```python
from build123d import *
from build123d.topology import SkipClean

# Parameters (mm, degrees)
SKETCH9_W            = 36
SKETCH9_H            = 36
BOSS_EXTRUDE1_DEPTH  = 40
CHAMFER2_SIZE        = 18
SKETCH10_W           = 36
SKETCH10_H           = 40
BOSS_EXTRUDE2_DEPTH  = 8
SKETCH12_W           = 44
SKETCH12_H           = 40
BOSS_EXTRUDE3_DEPTH  = 8
CHAMFER3_SIZE        = 18
CHAMFER4_SIZE        = 6
SKETCH13_W           = 36.769552622
SKETCH13_H           = 20
CUT_EXTRUDE6_DEPTH   = 39.59798
SKETCH22_R           = 2.1
CUT_EXTRUDE13_DEPTH  = 6
BOSS_EXTRUDE7_DEPTH  = 8
BOSS_EXTRUDE8_DEPTH  = 12
BOSS_EXTRUDE9_DEPTH  = 4
CUT_EXTRUDE14_DEPTH  = 4
CUT_EXTRUDE15_DEPTH  = 4
SKETCH28_W           = 4
SKETCH28_H           = 28
CUT_EXTRUDE16_DEPTH  = 77.210235533
BOSS_EXTRUDE11_DEPTH = 28
SKETCH31_W           = 10
SKETCH31_H           = 36
CUT_EXTRUDE17_DEPTH  = 22
SKETCH32_W           = 44
SKETCH32_H           = 18.026894841
CUT_EXTRUDE18_DEPTH  = 72.888803022
BOSS_EXTRUDE12_DEPTH = 10
BOSS_EXTRUDE13_DEPTH = 10
CHAMFER5_SIZE        = 6
CUT_EXTRUDE19_DEPTH  = 79.409183136
CHAMFER6_SIZE        = 6
SKETCH37_R           = 2.8
CUT_EXTRUDE20_DEPTH  = 7
BOSS_EXTRUDE14_DEPTH = 14
CHAMFER7_SIZE        = 14
CHAMFER8_SIZE        = 4
BOSS_EXTRUDE15_START = 7
SKETCH41_R           = 2.8
BOSS_EXTRUDE15_DEPTH = 7
BOSS_EXTRUDE16_START = 7
SKETCH42_R           = 2.8
BOSS_EXTRUDE16_DEPTH = 7
CHAMFER9_SIZE        = 1
SKETCH43_R           = 2.25
CUT_EXTRUDE21_DEPTH  = 69.381283989
SKETCH44_R           = 4
CUT_EXTRUDE22_DEPTH  = 7
CHAMFER11_SIZE       = 4
CHAMFER12_SIZE       = 3
SKETCH48_R           = 2.1
CUT_EXTRUDE26_DEPTH  = 4
SKETCH49_R           = 2.1
CUT_EXTRUDE27_DEPTH  = 4
CUT_EXTRUDE28_DEPTH  = 79.409183136


with BuildPart() as part:
    # Sketch9 → Boss-Extrude1 (new body)
    with BuildSketch(Plane(origin=(0, 0, 0), x_dir=(1, 0, 0), z_dir=(0, 1, 0))):
        with Locations((18, 18)):
            Rectangle(SKETCH9_W, SKETCH9_H)
    extrude(amount=BOSS_EXTRUDE1_DEPTH)

    # Chamfer2
    chamfer2_edges = [part.edges().sort_by_distance(p)[0] for p in [
        (0, 20, -36),
    ]]
    chamfer(chamfer2_edges, length=CHAMFER2_SIZE)

    # Sketch10 → Boss-Extrude2 (add)
    with BuildSketch(Plane(origin=(36, 0, 0), x_dir=(0, 0, -1), z_dir=(1, 0, 0))):
        with Locations((18, 20)):
            Rectangle(SKETCH10_W, SKETCH10_H)
    extrude(amount=BOSS_EXTRUDE2_DEPTH)

    # Sketch12 → Boss-Extrude3 (add)
    with BuildSketch(Plane.XY):
        with Locations((22, 20)):
            Rectangle(SKETCH12_W, SKETCH12_H)
    extrude(amount=BOSS_EXTRUDE3_DEPTH)

    # Chamfer3
    chamfer3_edges = [part.edges().sort_by_distance(p)[0] for p in [
        (44, 20, -36),
        (0, 20, 8),
    ]]
    chamfer(chamfer3_edges, length=CHAMFER3_SIZE)

    # Chamfer4
    chamfer4_edges = [part.edges().sort_by_distance(p)[0] for p in [
        (44, 20, 8),
    ]]
    chamfer(chamfer4_edges, length=CHAMFER4_SIZE)

    # Sketch13 → Cut-Extrude6 (cut)
    with BuildSketch(Plane(origin=(23, 0, 23), x_dir=(0.7071067811865465, 0, -0.7071067811865487), z_dir=(0.7071067811865487, 0, 0.7071067811865465))):
        with Locations((25.455844123, 22)):
            Rectangle(SKETCH13_W, SKETCH13_H)
    extrude(amount=-CUT_EXTRUDE6_DEPTH, mode=Mode.SUBTRACT)

    # Sketch22 → Cut-Extrude13 (cut)
    with BuildSketch(Plane(origin=(-9, 0, -9), x_dir=(-0.7071067811865487, 0, 0.7071067811865465), z_dir=(-0.7071067811865465, 0, -0.7071067811865487))):
        with Locations((-15.455844123, 36)):
            Circle(SKETCH22_R)
        with Locations((-35.455844123, 36)):
            Circle(SKETCH22_R)
        with Locations((-35.455844123, 4)):
            Circle(SKETCH22_R)
        with Locations((-15.455844123, 4)):
            Circle(SKETCH22_R)
    extrude(amount=-CUT_EXTRUDE13_DEPTH, mode=Mode.SUBTRACT)

    # Sketch23 → Boss-Extrude7 (add)
    with BuildSketch(Plane(origin=(0, 40, 0), x_dir=(1, 0, 0), z_dir=(0, 1, 0))):
        Polygon((26, 36), (44, 36), (44, 18), align=None)
    extrude(amount=-BOSS_EXTRUDE7_DEPTH)

    # Sketch24 → Boss-Extrude8 (add)
    with BuildSketch(Plane(origin=(0, 0, 0), x_dir=(-1, 0, 0), z_dir=(0, -1, 0))):
        Polygon((-44, 18), (-26, 36), (-44, 36), align=None)
    extrude(amount=-BOSS_EXTRUDE8_DEPTH)

    # Sketch25 → Boss-Extrude9 (add)
    with BuildSketch(Plane(origin=(0, 40, 0), x_dir=(1, 0, 0), z_dir=(0, 1, 0))):
        Polygon((18, -8), (38, -8), (44, -2), (44, 36), (18, 36), (0, 18), (0, 10), align=None)
    extrude(amount=BOSS_EXTRUDE9_DEPTH)

    # Sketch26 → Cut-Extrude14 (cut)
    with SkipClean():  # the faces are left unmerged after this step: merging them gives an invalid solid
        with BuildSketch(Plane(origin=(0, 32, 0), x_dir=(-1, 0, 0), z_dir=(0, -1, 0))):
            Polygon((-44, 36), (-44, -2), (-38, -8), (-18, -8), (0, 10), (-26, 36), align=None)
        extrude(amount=-CUT_EXTRUDE14_DEPTH, mode=Mode.SUBTRACT)

    # Sketch27 → Cut-Extrude15 (cut)
    with BuildSketch(Plane(origin=(0, 12, 0), x_dir=(1, 0, 0), z_dir=(0, 1, 0))):
        Polygon((44, -2), (44, 36), (26, 36), (0, 10), (18, -8), (38, -8), align=None)
    extrude(amount=-CUT_EXTRUDE15_DEPTH, mode=Mode.SUBTRACT)

    # Sketch28 → Cut-Extrude16 (cut, through all)
    with BuildSketch(Plane(origin=(0, 0, -36), x_dir=(-1, 0, 0), z_dir=(0, 0, -1))):
        with Locations((-24, 22)):
            Rectangle(SKETCH28_W, SKETCH28_H)
    extrude(amount=-CUT_EXTRUDE16_DEPTH, mode=Mode.SUBTRACT)

    # Sketch30 → Boss-Extrude11 (add)
    with BuildSketch(Plane(origin=(0, 8, 0), x_dir=(1, 0, 0), z_dir=(0, 1, 0))):
        Polygon((0, 10), (22, 10), (22, 32), align=None)
    extrude(amount=BOSS_EXTRUDE11_DEPTH)

    # Sketch31 → Cut-Extrude17 (cut)
    with BuildSketch(Plane(origin=(44, 0, 0), x_dir=(0, 0, -1), z_dir=(1, 0, 0))):
        with Locations((24, 22)):
            Rectangle(SKETCH31_W, SKETCH31_H)
    extrude(amount=-CUT_EXTRUDE17_DEPTH, mode=Mode.SUBTRACT)

    # Sketch32 → Cut-Extrude18 (cut, through all)
    with BuildSketch(Plane(origin=(0, 0, 0), x_dir=(-1, 0, 0), z_dir=(0, -1, 0))):
        with Locations((-22, 0.986552579)):
            Rectangle(SKETCH32_W, SKETCH32_H)
    extrude(amount=-CUT_EXTRUDE18_DEPTH, mode=Mode.SUBTRACT)

    # Sketch33 → Boss-Extrude12 (add)
    with BuildSketch(Plane(origin=(44, 0, 0), x_dir=(0, 0, -1), z_dir=(1, 0, 0))):
        Polygon((10, 8), (10, 0), (36, 0), (36, 8), (29, 8), (29, 4), (19, 4), (19, 8), align=None)
    extrude(amount=BOSS_EXTRUDE12_DEPTH)

    # Sketch35 → Boss-Extrude13 (add)
    with BuildSketch(Plane(origin=(44, 0, 0), x_dir=(0, 0, -1), z_dir=(1, 0, 0))):
        Polygon((10, 44), (10, 36), (19, 36), (19, 40), (29, 40), (29, 36), (36, 36), (36, 44), align=None)
    extrude(amount=BOSS_EXTRUDE13_DEPTH)

    # Chamfer5
    chamfer5_edges = [part.edges().sort_by_distance(p)[0] for p in [
        (54, 4, -10),
        (54, 4, -36),
        (54, 40, -10),
        (54, 40, -36),
    ]]
    chamfer(chamfer5_edges, length=CHAMFER5_SIZE)

    # Sketch36 → Cut-Extrude19 (cut, through all)
    with BuildSketch(Plane(origin=(0, 44, 0), x_dir=(1, 0, 0), z_dir=(0, 1, 0))):
        Polygon((14, 32), (14, 26), (10, 22), (4, 22), align=None)
    extrude(amount=-CUT_EXTRUDE19_DEPTH, mode=Mode.SUBTRACT)

    # Chamfer6
    chamfer6_edges = [part.edges().sort_by_distance(p)[0] for p in [
        (22, 22, -10),
    ]]
    chamfer(chamfer6_edges, length=CHAMFER6_SIZE)

    # Sketch37 → Cut-Extrude20 (cut)
    with BuildSketch(Plane(origin=(22, 0, 0), x_dir=(0, 0, -1), z_dir=(1, 0, 0))):
        with Locations(Location((24, 31, 0), (0, 0, 90))):
            Circle(SKETCH37_R)
        with Locations(Location((24, 13, 0), (0, 0, 90))):
            Circle(SKETCH37_R)
    extrude(amount=-CUT_EXTRUDE20_DEPTH, mode=Mode.SUBTRACT)

    # Sketch39 → Boss-Extrude14 (add)
    with BuildSketch(Plane.XY.offset(-10)):
        Polygon((48, 8), (16, 8), (16, 36), (48, 36), (48, 44), (0, 44), (0, 0), (48, 0), align=None)
    extrude(amount=BOSS_EXTRUDE14_DEPTH)

    # Chamfer7
    chamfer7_edges = [part.edges().sort_by_distance(p)[0] for p in [
        (48, 4, 4),
        (48, 40, 4),
    ]]
    chamfer(chamfer7_edges, length=CHAMFER7_SIZE - 0.0001)  # a hair under: the kernel refuses the full size

    # Chamfer8
    chamfer8_edges = [part.edges().sort_by_distance(p)[0] for p in [
        (17.00005, 0, 4),
        (0, 22, 4),
        (17.00005, 44, 4),
        (41.00005, 0, -2.99995),
        (48, 0, -9.99995),
        (51, 0, -13),
        (41.00005, 44, -2.99995),
        (48, 44, -9.99995),
        (51, 44, -13),
    ]]
    chamfer(chamfer8_edges, length=CHAMFER8_SIZE)

    # Sketch41 → Boss-Extrude15 (add)
    with BuildSketch(Plane(origin=(15, 0, 0), x_dir=(0, 0, -1), z_dir=(1, 0, 0)).offset(BOSS_EXTRUDE15_START)):
        with Locations((24, 31)):
            Circle(SKETCH41_R)
    extrude(amount=-BOSS_EXTRUDE15_DEPTH)

    # Sketch42 → Boss-Extrude16 (add)
    with BuildSketch(Plane(origin=(15, 0, 0), x_dir=(0, 0, -1), z_dir=(1, 0, 0)).offset(BOSS_EXTRUDE16_START)):
        with Locations((24, 13)):
            Circle(SKETCH42_R)
    extrude(amount=-BOSS_EXTRUDE16_DEPTH)

    # Chamfer9
    chamfer9_edges = [part.edges().sort_by_distance(p)[0] for p in [
        (54, 6, -29),
        (54, 4, -24),
        (54, 6, -19),
        (54, 38, -19),
        (54, 40, -24),
        (54, 38, -29),
    ]]
    chamfer(chamfer9_edges, length=CHAMFER9_SIZE - 0.0001)  # a hair under: the kernel refuses the full size

    # Sketch43 → Cut-Extrude21 (cut, through all)
    with BuildSketch(Plane(origin=(16, 0, 0), x_dir=(0, 0, -1), z_dir=(1, 0, 0))):
        with Locations(Location((3, 22, 0), (0, 0, 90))):
            Circle(SKETCH43_R)
    extrude(amount=-CUT_EXTRUDE21_DEPTH, mode=Mode.SUBTRACT)

    # Sketch44 → Cut-Extrude22 (cut)
    with BuildSketch(Plane.ZY):
        with Locations((-3, 22)):
            Circle(SKETCH44_R)
    extrude(amount=-CUT_EXTRUDE22_DEPTH, mode=Mode.SUBTRACT)

    # Chamfer10: read off the stored shape, not the designer's step
    # Chamfer10 outline → Chamfer10 (revolve, cut)
    with BuildSketch(Plane(origin=(0, 22, -3), x_dir=(0, 1, 0), z_dir=(0, 0, -1))):
        Polygon((8, 0), (4, 4), (4, 0), align=None)
    revolve(axis=Axis((0, 22, -3), (1, 0, 0)), mode=Mode.SUBTRACT)

    # Chamfer11
    chamfer11_edges = [part.edges().sort_by_distance(p)[0] for p in [
        (0, 44, -9),
    ]]
    chamfer(chamfer11_edges, length=CHAMFER11_SIZE)

    # Chamfer12
    chamfer12_edges = [part.edges().sort_by_distance(p)[0] for p in [
        (0, 0, -9),
    ]]
    chamfer(chamfer12_edges, length=CHAMFER12_SIZE)

    # Sketch48 → Cut-Extrude26 (cut)
    with BuildSketch(Plane(origin=(0, 0, 0), x_dir=(-1, 0, 0), z_dir=(0, -1, 0))):
        with Locations(Location((-28.025270862, 18.024920623, 0), (0, 0, 90))):
            Circle(SKETCH48_R)
        with Locations(Location((-18.025270862, 8.024920623, 0), (0, 0, 90))):
            Circle(SKETCH48_R)
    extrude(amount=-CUT_EXTRUDE26_DEPTH, mode=Mode.SUBTRACT)

    # Sketch49 → Cut-Extrude27 (cut)
    with BuildSketch(Plane(origin=(0, 44, 0), x_dir=(1, 0, 0), z_dir=(0, 1, 0))):
        with Locations(Location((17.898400733, 7.868441876, 0), (0, 0, 270))):
            Circle(SKETCH49_R)
        with Locations(Location((27.898400733, 17.868441876, 0), (0, 0, 270))):
            Circle(SKETCH49_R)
    extrude(amount=-CUT_EXTRUDE27_DEPTH, mode=Mode.SUBTRACT)

    # Sketch50 → Cut-Extrude28 (cut, through all)
    with BuildSketch(Plane(origin=(0, 0, 0), x_dir=(-1, 0, 0), z_dir=(0, -1, 0))):
        Polygon((-3.535533906, 21.535533906), (-10.928932188, 21.535533906), (-14.464466094, 25.071067812), (-14.464466094, 32.464466094), align=None)
    extrude(amount=-CUT_EXTRUDE28_DEPTH, mode=Mode.SUBTRACT)


solid = part.part
```
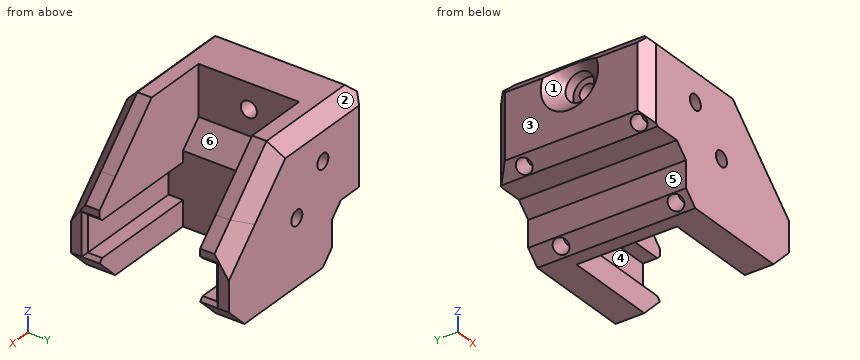
Model file for the job. Use its own axes, mm. Face numbers are marked on the shaded views. A direction names the side the tool comes from. Coordinates: 2 decimals unless noted, no trailing zeros. Order: outer loops, then holes, each group sorted by start corner. A loop starts at its lowest first (then second) coordinate and runs counter-clockwise, first axis right, second up. Notation, with made-up numbers: (51.5, 19) -> (105.5, 19) arc R23 ccw to (105.5, 37) -> close; hole circle Ø9 at (-18, 43). An arc over 180 degrees is marked (long way). Return JSON: item names as keys, results as strings.
Item 1: Slice it at A-A (x = 9). Write the cut outline in (y, z).
Model answer:
{"outline": "(0, -21.54) -> (44, -21.54) -> (44, 0) -> (40, 4) -> (4, 4) -> (0, 0) -> close; hole circle Ø4.5 at (22, -3)"}
Item 2: Slice it at B-B (y = 22). Write the cut outline in (x, z).
Model answer:
{"outline": "(0, -18) -> (3.54, -21.54) -> (10.93, -21.54) -> (14.46, -25.07) -> (14.46, -32.46) -> (18, -36) -> (22, -36) -> (22, -16) -> (16, -10) -> (16, -5.25) -> (7, -5.25) -> (7, -7) -> (4, -7) -> (0, -11) -> close; (2.5, 2.5) -> (4, 1) -> (7, 1) -> (7, -0.75) -> (16, -0.75) -> (16, 4) -> (4, 4) -> close"}
Item 3: Slice it at C-C (x = 25). Write the cut outline in (y, z).
Model answer:
{"outline": "(0, -36) -> (8, -36) -> (8, -29) -> (4, -29) -> (4, -19) -> (8, -19) -> (8, 4) -> (4, 4) -> (0, 0) -> close; (36, -36) -> (44, -36) -> (44, 0) -> (40, 4) -> (36, 4) -> (36, -19) -> (40, -19) -> (40, -29) -> (36, -29) -> close"}
Item 4: Slice it at D-D (z = -3). Write the cut outline in (x, y).
Model answer:
{"outline": "(0, 3) -> (3, 0) -> (35.34, 0) -> (41, 4) -> (41, 8) -> (16, 8) -> (16, 19.75) -> (7, 19.75) -> (7, 18) -> (4, 18) -> (0, 14) -> close; (0, 30) -> (4, 26) -> (7, 26) -> (7, 24.25) -> (16, 24.25) -> (16, 36) -> (41, 36) -> (41, 40) -> (35.34, 44) -> (4, 44) -> (0, 40) -> close"}
Item 5: Mould opens along Z. For the marked faces 1, 2 and 3 say: pulls with the +Z half, pulls with the -Z half, needs draft (parallel to the pull), parting line crosses it, or undercut.
Model answer:
{"face 1": "undercut", "face 2": "pulls with the +Z half", "face 3": "needs draft"}
Item 6: 3-axis set-ups, long thin cutter, end or side, ignore diameter. For the marked faces 4, 5 and 6: which of +Z, -Z, +X, -X, +Y, -Y reach the whole face in a straight line?
Model answer:
{"face 4": "+X", "face 5": "-Z, -X, +Y, -Y", "face 6": "+Z, +X"}
Item 7: Wall check: line 1 along Y through (x, z) = (41.5, -14.5); line 2 along Z through (x, y) = (24, 5.5); line 3 along X through (y, z) = (18, -16.5). Give the ranges that are in metal, low to high. Write a range as from..to.
Model answer:
{"line 1": "y = 0..8, 36..44", "line 2": "z = -36..-29, -19..4", "line 3": "x = 0..22"}
Item 8: Pin check, flat tips, straight feed: P1, Ø9, axis at y = 21.5, z = -5, coming from the -X side; P2, Ø15.5, axis at y = 22, z = -1.5, coming from the +X side; P3, Ø6, axis at y = 19, z = -26.5, coming from the +X side. Stop position of each tip, or through.
Model answer:
{"P1": "stops at x = 1.44", "P2": "stops at x = 16", "P3": "stops at x = 22"}
